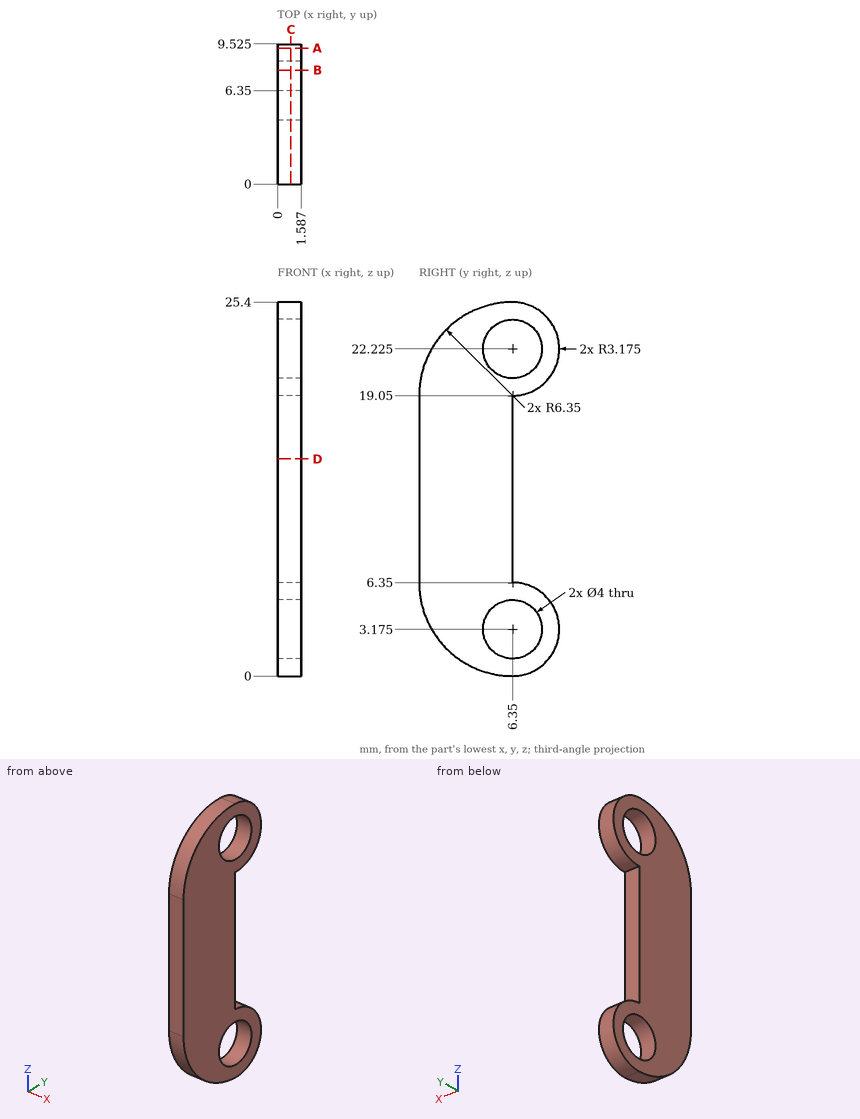
Geometry: see drawing. Coordinates: mm, zero at the bounding-box minimum. Give positions to 0.01 mm unless a question says otherwise; leave off trailing zeros. Order: outer loops, then holes, each group sorted by start corner. A loop starts at its lowest first (then second) coordinate and runs counter-clockwise, first axis right, second up.
1. Line query: probe 1 along Z at (x, y) = (0.8, 8) (1 decimal); probe 2 along Z at (x, y) = (1, 6) (1 decimal); probe 3 along Z at (x, y) = (0.85, 7.5) (1 decimal). Output: solid intervals per line, ascending.
Computed:
probe 1: z = 0.5 to 2, 4.3 to 5.9, 19.5 to 21.1, 23.4 to 24.9
probe 2: z = 0 to 1.2, 5.1 to 20.3, 24.2 to 25.4
probe 3: z = 0.2 to 1.5, 4.8 to 6.1, 19.3 to 20.6, 23.9 to 25.2
2. Cut plane D-D (z = 14.75). Return loops of the section in (x, y), and give its area (3 significant figures).
Computed:
outline: (0, 0) - (1.59, 0) - (1.59, 6.35) - (0, 6.35) - close
area: 10.1 mm2
3. Cut plane C-C (x = 0.9). State how many separate pieces and enclosed holes the cut face has.
Computed:
separate pieces: 1
enclosed holes: 2
4. Cut plane B-B (y = 7.75). Return loops of the section in (x, z) (1 decimal).
Computed:
outline: (0, 0.3) - (1.6, 0.3) - (1.6, 1.7) - (0, 1.7) - close; (0, 4.6) - (1.6, 4.6) - (1.6, 6) - (0, 6) - close; (0, 19.4) - (1.6, 19.4) - (1.6, 20.8) - (0, 20.8) - close; (0, 23.7) - (1.6, 23.7) - (1.6, 25.1) - (0, 25.1) - close
5. Pin query (flat end, axial travel): pin 1 Ø0.8 at (x, z) = (1, 9.5) entering from +Y. Return the tip coordinate at first contact, or that it passes through.
Computed:
pin 1: stops at y = 6.35
6. Cut plane A-A (y = 9.25). Return loops of the section in (x, z).
Computed:
outline: (0, 1.88) - (1.59, 1.88) - (1.59, 4.47) - (0, 4.47) - close; (0, 20.93) - (1.59, 20.93) - (1.59, 23.52) - (0, 23.52) - close
